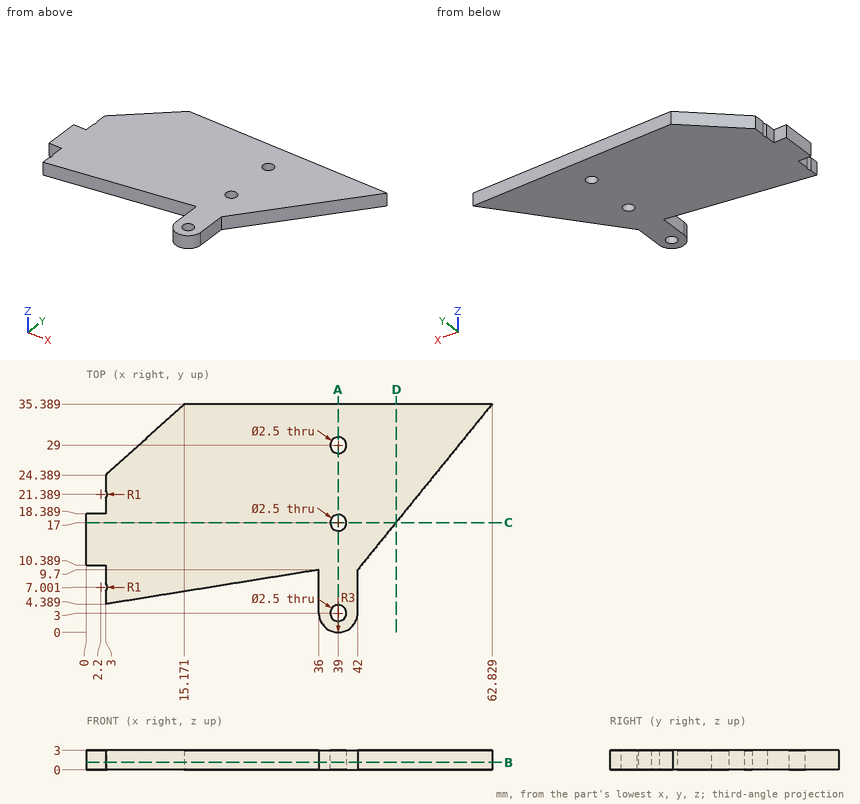
Study the drawing (mm; zero at the part's minimum x, y, z) and answer. Give positions to 0.01 mm unless a question says otherwise; leave off trailing zeros. Order: outer loops, then holes, each group sorted by start corner. A loop starts at its lowest first (then second) coordinate and runs counter-clockwise, first axis right, second up.
1. Section A-A, the plane x = 39 is taken. Determine the outline of the cut face in (y, z), and give its area (3 significant figures).
Result sheet:
outline: (0, 0) - (1.75, 0) - (1.75, 3) - (0, 3) - close; (4.25, 0) - (15.75, 0) - (15.75, 3) - (4.25, 3) - close; (18.25, 0) - (27.75, 0) - (27.75, 3) - (18.25, 3) - close; (30.25, 0) - (35.39, 0) - (35.39, 3) - (30.25, 3) - close
area: 83.7 mm2
2. Section B-B, the plane z = 1.15 is taken. Determine the outline of the cut face in (x, y), and give its area (3 significant figures).
Result sheet:
outline: (0, 10.39) - (3, 10.39) - (3, 7.6) arc R1 cw to (3, 6.4) - (3, 4.39) - (36, 9.7) - (36, 3) arc R3 ccw to (42, 3) - (42, 9.7) - (62.83, 35.39) - (15.17, 35.39) - (3, 24.39) - (3, 21.99) arc R1 cw to (3, 20.79) - (3, 18.39) - (0, 18.39) - close; hole circle Ø2.5 at (39, 3); hole circle Ø2.5 at (39, 17); hole circle Ø2.5 at (39, 29)
area: 1,350 mm2
3. Section D-D, the plane x = 48 is taken. Determine the outline of the cut face in (y, z), and give its area (3 significant figures).
Result sheet:
outline: (17.1, 0) - (35.39, 0) - (35.39, 3) - (17.1, 3) - close
area: 54.9 mm2
4. Straight lines are drawn through the part: L1, parallel to Y at x = 39, z = 1.4; L2, parallel to Y at x = 51, z = 0.65; L3, parallel to X at y = 16.5, z = 0.8. For each, find the intervals that lie inside material, in ascending order.
Result sheet:
L1: y = 0 to 1.75, 4.25 to 15.75, 18.25 to 27.75, 30.25 to 35.39
L2: y = 20.8 to 35.39
L3: x = 0 to 37.85, 40.15 to 47.51
5. Each of these flat-tipped pins is pushed along its axis until it touches: P1, Ø1.5, axis at x = 1, z = 1, coming from the -Y side; P2, Ø1.6, axis at y = 5, z = 2, coming from the -X side; P3, Ø1, axis at x = 12, z = 0.5, coming from the -Y side. Where does it stop, or does it pass through?
Result sheet:
P1: stops at y = 10.39
P2: stops at x = 3
P3: stops at y = 5.76
6. Section C-C, the plane y = 17 is taken. Determine the outline of the cut face in (x, z), and give its area (3 significant figures).
Result sheet:
outline: (0, 0) - (37.75, 0) - (37.75, 3) - (0, 3) - close; (40.25, 0) - (47.92, 0) - (47.92, 3) - (40.25, 3) - close
area: 136 mm2
